```python
from build123d import *

# Parameters (mm, degrees)
F1_DEPTH = 2.54
F2_SIZE  = 2.032
F3_SCALE = 1.2


with BuildPart() as f1:
    # F0 (on Top) → F1 (new body)
    with BuildSketch(Plane.XY):
        with BuildLine():
            Line((4.7955396725, 11.2255265503), (0, 44.45))
            Line((0, 44.45), (-4.7955396725, 11.2255265503))
            Line((-4.7955396725, 11.2255265503), (-16.326805286, 19.4575288552))
            Line((-16.326805286, 19.4575288552), (-7.0366641055, 0))
            Line((-7.0366641055, 0), (-16.326805286, -19.4575288552))
            Line((-16.326805286, -19.4575288552), (-2.0887149606, -9.2931638753))
            ThreePointArc((-2.0887149606, -9.2931638753), (-1.5548922201, -9.3972301868), (-1.016, -9.4706583193))
            Line((-1.016, -9.4706583193), (-1.016, -11.2221352642))
            ThreePointArc((-1.016, -11.2221352642), (0, -20.6375), (1.016, -11.2221352642))
            Line((1.016, -11.2221352642), (1.016, -9.4706583193))
            ThreePointArc((1.016, -9.4706583193), (1.5548922201, -9.3972301868), (2.0887149606, -9.2931638753))
            Line((2.0887149606, -9.2931638753), (16.326805286, -19.4575288552))
            Line((16.326805286, -19.4575288552), (7.0366641055, 0))
            Line((7.0366641055, 0), (16.326805286, 19.4575288552))
            Line((16.326805286, 19.4575288552), (4.7955396725, 11.2255265503))
        make_face()
    extrude(amount=F1_DEPTH)

    # F2
    f2_edges = [f1.edges().sort_by_distance(p)[0] for p in [
        (-2.39777, 27.837763, 2.54),
        (10.561172, 15.341528, 2.54),
        (11.681735, 9.728764, 2.54),
        (-10.561172, 15.341528, 2.54),
        (-11.681735, 9.728764, 2.54),
        (2.39777, 27.837763, 2.54),
        (11.681735, -9.728764, 2.54),
        (9.20776, -14.375346, 2.54),
        (-9.20776, -14.375346, 2.54),
        (-11.681735, -9.728764, 2.54),
        (0, -20.6375, 2.54),
    ]]
    chamfer(f2_edges, length=F2_SIZE)


with BuildPart() as f1_1:
    # F3: moved
    add(f1.part.scale(F3_SCALE))


solid = f1_1.part
```
The model under review builds one solid part; all positions refer to its coordinate system, in mm. A direction names the side the tool comes from. Round coordinates to 2 decimals unless told otherwise and drop trailing zeros. Loops run counter-clockwise (first coordinate to the right, second up) from the corner with the lowest first, then second, coordinate; pieces in that order, holes last. Notation, with made-up numbers: (66.25, -40) - (111.25, -40) arc R28 cw to (111.25, -9) - close; hole circle Ø8 at (-4.5, 6). An arc over 180 degrees is marked (long way). Write each question's results on one line, items separated by ' | '. Start each with the question number.
Q1. Take a section at D-D on x = 10. Give the boundary of the cut face in (y, z), plus the area to 3 significant figures.
Q2. Take a section at B-B on y = -19.05. Give the boundary of the cut face in (x, z) (3 decimals).
Q3. Draft analysis for pull direction Y (two halves, no side actions). For faces 4 (the cylindrical face through (2.822, -11.076, 1.841)), 5 (the flat face through (0, 1, 3.048)), 6 (the flat face through (12.8, 18.5, 0.3)), state which applies: pulls with the +Y half, pulls with the -Y half, needs draft (parallel to the pull), parting line crosses it, or undercut.
Q4. Tool access review of faces 1 (the flat face through (-11.169, -17.336, 0.301)), 2 (the flat face through (-12.577, 18.341, 0.301)), 3 (the flat face through (11.276, 8.8, 1.846)): name each direction out of +Z, -Z, +X, -X, +Y, -Y from which nothing blocks a thin tool from reaching the whole face with its end or side.
Q5. Insertion check: P1, Ø12, axis at x = -4.5, y = 20, coming from the -Z side; P2, Ø1.5, axis at y = -13, z = 2, coming from the -X side. Each pin has a flat end and moves straight along its axis. Give the tip position at first contact, or say it passes through.
Q6. Wall thickness on line 1 along X through (y, z) = (-16, 1.05); line 2 along X through (y, z) = (-15.5, 0.55); line 3 along Y through (x, z) = (-11.5, 1.75): over which ranges is each line inside the solid? List them lowest first. Write a range as [from, to].
Q7. Take a section at C-C on z = 2.05. Give the boundary of the cut face in (x, y), plus the area to 3 significant figures.
Q8. Take a section at A-A on x = -15.5. Give the boundary of the cut face in (y, z).
Data:
1) outline: (-16.5, 0) - (-3.26, 0) - (-3.26, 0.61) - (-8.92, 3.05) - (-13.51, 3.05) - (-16.5, 0.61) - close; (3.26, 0) - (16.5, 0) - (16.5, 0.61) - (13.51, 3.05) - (8.92, 3.05) - (3.26, 0.61) - close | area: 59.6 mm²
2) outline: (-17.54, 0) - (-13.57, 0) - (-13.57, 0.61) - (-15.985, 2.013) - (-17.54, 0.61) - close; (-5.715, 0) - (5.715, 0) - (5.715, 0.61) - (3.277, 3.048) - (-3.277, 3.048) - (-5.715, 0.61) - close; (13.57, 0) - (17.54, 0) - (17.54, 0.61) - (15.985, 2.013) - (13.57, 0.61) - close
3) face 4: undercut | face 5: needs draft | face 6: pulls with the +Y half
4) face 1: +Z, -Z | face 2: +Z, -Z, +Y | face 3: +Z, +X
5) P1: stops at z = 0 | P2: stops at x = -14.02
6) line 1: x = [-15.6, -10.06], [-4.3, 4.3], [10.06, 15.6] | line 2: x = [-15.84, -8.6], [-4.48, 4.48], [8.6, 15.84] | line 3: y = [-16.17, -9.05], [9.05, 16.17]
7) outline: (-15.89, -18.94) - (-4.24, -10.62) arc R11.43 ccw to (-1.22, -11.36) - (-1.22, -14.95) arc R4.27 ccw (long way) to (1.22, -14.95) - (1.22, -11.36) arc R11.43 ccw to (4.24, -10.62) - (15.89, -18.94) - (6.85, 0) - (15.89, 18.94) - (4.67, 10.92) - (0, 43.26) - (-4.67, 10.92) - (-15.89, 18.94) - (-6.85, 0) - close | area: 750 mm²
8) outline: (-20.43, 0) - (-14.78, 0) - (-14.78, 0.61) - (-18.47, 2.2) - (-20.43, 0.61) - close; (14.78, 0) - (20.43, 0) - (20.43, 0.61) - (18.47, 2.2) - (14.78, 0.61) - close
